Autodesk Inventor part; units mm, degrees
ref_plane "YZ Plane" through (0, 0, 0) normal (1, 0, 0) x (0, 1, 0)
ref_plane "XZ Plane" through (0, 0, 0) normal (0, 1, 0) x (-1, 0, 0)
ref_plane "XY Plane" through (0, 0, 0) normal (0, 0, 1) x (1, 0, 0)
sketch "Sketch1" plane through (0, 0, 0) normal (0, 0, 1) x (1, 0, 0)
  circle A0 centre (0, 0) radius 20
  dimension "d0" = 40
extrude "Extrusion1" add sketch "Sketch1" along normal blind 24
sketch "Sketch2" plane through (0, 0, 24) normal (0, 0, 1) x (1, 0, 0)
  arc A0 (-9.5263, 5.5) -> (-9.5263, -5.5) centre (0, 0) ccw
  line L0 (-9.5263, 5.5) -> (-17.3205, 10)
  circle A1 centre (0, 0) radius 20
  line L1 (0, 0) -> (20, 0) construction
  line L2 (-9.5263, -5.5) -> (-17.3205, -10)
  line L3 (0, 0) -> (20, 0) construction
  line L4 (0, 0) -> (0, 20) construction
  arc A2 (9.5263, -5.5) -> (9.5263, 5.5) centre (0, 0) ccw
  line L5 (9.5263, 5.5) -> (17.3205, 10)
  line L6 (9.5263, -5.5) -> (17.3205, -10)
  dimension "d3" = 22
  dimension "d4" = 150
  dimension "d5" = 150
extrude "Extrusion2" add sketch "Sketch2" along normal blind 13 contours A0 L2 A1 L0 | A1 L6 A2 L5
sketch "Sketch3" plane through (0, 0, 24) normal (0, 0, 1) x (1, 0, 0)
  circle A0 centre (0, 0) radius 10
  dimension "d8" = 20
extrude "Extrusion3" cut sketch "Sketch3" against normal through all
properties part number "LOWER-JAW"
Verification items for the finished model (mm, model axes). A direction names the side the tool comes from. Give positions to 0.01 mm unless a question says otherwise; leave off trailing zeros. Write each loop counter-clockwise with the first axis right and the second up, starting at its lowest first coordinate (ties: lowest second). Pieces come first, ordered by that corner, then holes.
(1) Cross-section at D-D (x = -13). Enter the section's corners in (y, z), plus the area to 3 significant figures.
(2) Material ranges on line 1 (Y direction, x = -0.5, z = 8); line 2 (Z direction, x = 11, y = 8.5); line 3 (Y direction, x = -7, z = 9.5) (3 decimals), recorded low to high.
(3) Cross-section at A-A (z = 31). Enter the section's corners in (x, y), plus the area to 3 significant figures.
(4) Mould release check, pull along X, two halves, no side actions. Record for faces 5 (the face through (13.37, -7.72, 30.41)), 6 (the face through (13.37, 7.72, 30.41)), 7 (the face through (-15, 0, 37)), 8 (the face through (7.6, 18.5, 14.1)): +X half, -X half, draft (parallel to the pull), parting line (faces both ways), or undercut.
(5) Gauge pin test, flat ends, axial feed: pin 1 (2 mm diameter, centred on y = 7, z = 17.5, fed in from -X); pin 2 (10 mm diameter, centred on x = -5.5, z = 9, fed in from -Y); pin 3 (6 mm diameter, centred on x = -8.5, z = 11.5, fed in from -Y). Record the tip position at first contact, or that the pin passes through.
(6) Cross-section at B-B (x = 0). Enter the section's corners in (y, z), plus the area to 3 significant figures.
(7) Access from +Z, -Z, +X, -X, +Y, -Y to the whole of each face (thin tool, end or side, straight path). Record for faces 1 (the face through (-13.37, -7.72, 30.41)), 2 (the face through (-13.37, 7.72, 30.41)), 3 (the face through (15, 0, 37)), 4 (the face through (11, 0, 30)).
(8) Cross-section at C-C (y = -8). Enter the section's corners in (x, z).
Worked out:
1. outline: (-15.2, 0) - (15.2, 0) - (15.2, 24) - (7.51, 24) - (7.51, 37) - (-7.51, 37) - (-7.51, 24) - (-15.2, 24) - close
1. area: 925 mm2
2. line 1: y = -19.99 to -9.99, 9.99 to 19.99
2. line 2: z = 0 to 24
2. line 3: y = -18.735 to -7.141, 7.141 to 18.735
3. outline: (-17.32, -10) - (-9.53, -5.5) arc R11 cw to (-9.53, 5.5) - (-17.32, 10) arc R20 ccw to start; (9.53, -5.5) - (17.32, -10) arc R20 ccw to (17.32, 10) - (9.53, 5.5) arc R11 cw to start
3. area: 292 mm2
4. face 5: undercut
4. face 6: undercut
4. face 7: draft
4. face 8: parting line
5. pin 1: stops at x = -19.08
5. pin 2: stops at y = -19.99
5. pin 3: stops at y = -19.23
6. outline: (-20, 0) - (-10, 0) - (-10, 24) - (-20, 24) - close; (10, 0) - (20, 0) - (20, 24) - (10, 24) - close
6. area: 480 mm2
7. face 1: +Z, -Y
7. face 2: +Z, +Y
7. face 3: +Z, +X, -X, +Y, -Y
7. face 4: +Z
8. outline: (-18.33, 0) - (-6, 0) - (-6, 24) - (-13.86, 24) - (-13.86, 37) - (-18.33, 37) - close; (6, 0) - (18.33, 0) - (18.33, 37) - (13.86, 37) - (13.86, 24) - (6, 24) - close
